Could you check a few things on this model? Use its own coordinates, in mm. A direction names the side the tool comes from. Give positions to 0.01 mm unless a question says otherwise; leave off trailing zeros. Loops run counter-clockwise (first coordinate to the right, second up) from the corner with the lowest first, then second, coordinate; pieces in that order, holes last.
1. Imagine slicing it at B-B (x = 0). List the corners of the cut face in (y, z) for me (3 decimals).
2. For faces 1 (the flat face through (15, 21, -13)), 2 (the cylindrical face through (47, 11, 4)), 3 (the flat face through (24.25, 2, 0)), which set-ups out of +Z, -Z, +X, -X, +Y, -Y let a thin tool reach every point of the face, with its end or its side?
3. Imagine slicing it at A-A (y = 27). List the corners of the cut face in (x, z) for me.
4. Imagine slicing it at C-C (z = 0). Count the separate pieces of the cut face and the enclosed holes in it, plus the area to 3 significant figures.
5. For P1, Ø13, axis at y = 17, z = 2.5, coming from the +X side; P2, Ø9, axis at x = 16, y = 20, coming from the -Z side; P3, Ø1.5, axis at y = 8, z = 6, coming from the +X side, each with a flat end and sliding along its axis, tell me the tip position at first contact or that it passes through.
6. Imagine slicing it at D-D (y = 14). List the corners of the cut face in (x, z) for me.
7. I need wall thicknesses on line 1 along Y through (x, z) = (15.5, -4.5); line 2 along Y through (x, z) = (47, 0); line 3 along X through (y, z) = (8, -8). Which ranges of each line are inside material? Lowest first, please.
8. Thinking about a two-plate mould opening in Z: for faces 4 (the flat face through (15, 5, 0)), 5 (the flat face through (50, 4, 0)), which applies, +Z half, -Z half, draft (parallel to the pull), parting line (faces both ways), or undercut?
```python
from build123d import *

# Parameters (mm, degrees)
SKETCH1_R               = 60.625
SKETCH1_R_2             = 45
BOSS_EXTRUDE1_DEPTH     = 4
SKETCH2_R               = 49
SKETCH2_R_2             = 45
BOSS_EXTRUDE2_DEPTH     = 52
SKETCH4_W               = 13.25
SKETCH4_H               = 8
SKETCH4_W_2             = 8
SKETCH4_H_2             = 38
BOSS_EXTRUDE4_DEPTH     = 13
BOSS_EXTRUDE5_DEPTH     = 4
SKETCH7_R               = 1.3
CUT_EXTRUDE4_DEPTH      = 7.2
SKETCH9_W               = 10
SKETCH9_H               = 24
CUT_EXTRUDE7_DEPTH      = 8
CUT_EXTRUDE8_REACH      = 139.219
CUT_EXTRUDE8_END_RADIUS = 45
SKETCH11_R              = 5
CUT_EXTRUDE9_DEPTH      = 101.273532203
SKETCH15_R              = 2.5
CUT_EXTRUDE10_DEPTH     = 10


with BuildPart() as part:
    # Sketch1 → Boss-Extrude1 (new body)
    with BuildSketch(Plane(origin=(0, 0, 0), x_dir=(1, 0, 0), z_dir=(0, 1, 0))):
        with Locations(Location((0, 0, 0), (0, 0, 270))):
            Circle(SKETCH1_R)
        with Locations(Location((0, 0, 0), (0, 0, 270))):
            Circle(SKETCH1_R_2, mode=Mode.SUBTRACT)
    extrude(amount=BOSS_EXTRUDE1_DEPTH)

    # Sketch2 → Boss-Extrude2 (add)
    with BuildSketch(Plane(origin=(0, 4, 0), x_dir=(1, 0, 0), z_dir=(0, 1, 0))):
        with Locations(Location((0, 0, 0), (0, 0, 90))):
            Circle(SKETCH2_R)
        with Locations(Location((0, 0, 0), (0, 0, 270))):
            Circle(SKETCH2_R_2, mode=Mode.SUBTRACT)
    extrude(amount=BOSS_EXTRUDE2_DEPTH)

    # Sketch4 → Boss-Extrude4 (add, symmetric)
    with BuildSketch(Plane.XY):
        with Locations((-38.375, 34)):
            Rectangle(SKETCH4_W, SKETCH4_H)
        Polygon((-31.75, 30), (-45, 30), (-45, 16.75), align=None)
        with Locations((15.25, 19)):
            Rectangle(SKETCH4_W_2, SKETCH4_H_2)
    extrude(amount=BOSS_EXTRUDE4_DEPTH, both=True)


with BuildPart() as boss_extrude4_piece_1:
    # of the separate pieces the step leaves, piece 1, a body of its own (boss_extrude4_pieces)
    add(part.part.solids().sort_by_distance((0, 0, 60.625))[0])



with BuildPart() as boss_extrude4_piece_2:
    # of the separate pieces the step leaves, piece 2, a body of its own (boss_extrude4_pieces)
    add(part.part.solids().sort_by_distance((11.25, 38, -13))[0])


with BuildPart() as boss_extrude4_piece_1_1:
    add(boss_extrude4_piece_1.part)

    add(boss_extrude4_piece_2.part)  # Boss-Extrude5 merges Boss-Extrude4 piece 2
    # Sketch5 → Boss-Extrude5 (add)
    with BuildSketch(Plane.XZ):
        with BuildLine():
            Line((11.25, 13), (29.067400866, 34.352382842))
            ThreePointArc((29.067400866, 34.352382842), (45, 0), (29.067400866, -34.352382842))
            Line((29.067400866, -34.352382842), (11.25, -13))
            Line((11.25, -13), (11.25, 13))
        make_face()
    extrude(amount=-BOSS_EXTRUDE5_DEPTH)

    # Sketch7 → Cut-Extrude4 (cut)
    with BuildSketch(Plane(origin=(0, 38, 0), x_dir=(1, 0, 0), z_dir=(0, 1, 0))):
        with Locations(Location((-34.25, 5, 0), (0, 0, 180))):
            Circle(SKETCH7_R)
        with Locations(Location((-34.25, -5, 0), (0, 0, 180))):
            Circle(SKETCH7_R)
        with Locations(Location((13.75, 5, 0), (0, 0, 180))):
            Circle(SKETCH7_R)
        with Locations(Location((13.75, -5, 0), (0, 0, 180))):
            Circle(SKETCH7_R)
    extrude(amount=-CUT_EXTRUDE4_DEPTH, mode=Mode.SUBTRACT)

    # Sketch9 → Cut-Extrude7 (cut)
    with BuildSketch(Plane.ZY.offset(-11.25)):
        with Locations((0, 17)):
            Rectangle(SKETCH9_W, SKETCH9_H)
    extrude(amount=-CUT_EXTRUDE7_DEPTH, mode=Mode.SUBTRACT)

    # Cut-Extrude8: up to this cylinder (the profile starts outside it)
    cut_extrude8_end = Plane(origin=(0, 14, 0), z_dir=(0, -1, 0)) * Cylinder(CUT_EXTRUDE8_END_RADIUS, 369.438, mode=Mode.PRIVATE)
    # Sketch11 → Cut-Extrude8 (cut, up to the surface)
    with BuildSketch(Plane(origin=(49, 0, 0), x_dir=(0, 0, -1), z_dir=(1, 0, 0)), mode=Mode.PRIVATE) as cut_extrude8_sk1:
        with Locations((0, 14)):
            Circle(SKETCH11_R)
    cut_extrude8_tool1 = extrude(cut_extrude8_sk1.sketch, amount=-CUT_EXTRUDE8_REACH, mode=Mode.PRIVATE) - cut_extrude8_end
    add(cut_extrude8_tool1.solids().sort_by_distance((49, 14, 0))[0], mode=Mode.SUBTRACT)

    # Sketch12 → Cut-Extrude9 (cut, through all)
    with BuildSketch(Plane(origin=(0, 4, 0), x_dir=(1, 0, 0), z_dir=(0, 1, 0))):
        with BuildLine():
            Line((29.479537487, 22.359715328), (27.25, 19.687836398))
            Line((27.25, 19.687836398), (27.25, -19.687836398))
            Line((27.25, -19.687836398), (29.479537487, -22.359715328))
            ThreePointArc((29.479537487, -22.359715328), (37, 0), (29.479537487, 22.359715328))
        make_face()
        Polygon((27.25, -19.687836398), (27.25, 19.687836398), (24.25, 16.092634774), (24.25, -16.092634774), align=None)
    extrude(amount=-CUT_EXTRUDE9_DEPTH, mode=Mode.SUBTRACT)

    # Sketch15 → Cut-Extrude10 (cut)
    with BuildSketch(Plane(origin=(0, 4, 0), x_dir=(1, 0, 0), z_dir=(0, 1, 0))):
        with Locations(Location((0, 55, 0), (0, 0, 270))):
            Circle(SKETCH15_R)
        with Locations(Location((52.308108396, 16.995934691, 0), (0, 0, 270))):
            Circle(SKETCH15_R)
        with Locations(Location((32.328188876, -44.495934691, 0), (0, 0, 270))):
            Circle(SKETCH15_R)
        with Locations(Location((-32.328188876, -44.495934691, 0), (0, 0, 270))):
            Circle(SKETCH15_R)
        with Locations(Location((-52.308108396, 16.995934691, 0), (0, 0, 270))):
            Circle(SKETCH15_R)
    extrude(amount=-CUT_EXTRUDE10_DEPTH, mode=Mode.SUBTRACT)


solid = boss_extrude4_piece_1_1.part
```
Derived:
1. outline: (0, -60.625) - (4, -60.625) - (4, -57.5) - (0, -57.5) - close; (0, -52.5) - (4, -52.5) - (4, -49) - (56, -49) - (56, -45) - (0, -45) - close; (0, 45) - (56, 45) - (56, 49) - (4, 49) - (4, 60.625) - (0, 60.625) - close
2. face 1: +Y
2. face 2: +X
2. face 3: +Y, -Y
3. outline: circle Ø98 at (0, 0); (11.25, -13) - (19.25, -13) - (19.25, -5) - (11.25, -5) - close; (11.25, 5) - (19.25, 5) - (19.25, 13) - (11.25, 13) - close; hole (-43.08, -13) arc R45 ccw (long way) to (-43.08, 13) - (-34.75, 13) - (-34.75, -13) - close
4. separate pieces: 5
4. enclosed holes: 0
4. area: 859 mm2
5. P1: stops at x = 49
5. P2: stops at z = -47.63
5. P3: stops at x = 48.72
6. outline: (11.25, -13) - (19.25, -13) - (19.25, -5) - (11.25, -5) - close; (11.25, 5) - (19.25, 5) - (19.25, 13) - (11.25, 13) - close; (44.72, -5) arc R45 cw (long way) to (44.72, 5) - (48.74, 5) arc R49 ccw (long way) to (48.74, -5) - close
7. line 1: y = 0 to 5, 29 to 38
7. line 2: y = 0 to 9, 19 to 56
7. line 3: x = -48.34 to -44.28, 11.25 to 19.25, 44.28 to 48.34
8. face 4: undercut
8. face 5: draft
